Geometry: final body of the model. Coordinates: model frame, mm. A direction names the side the tool comes from. Give positions to 0.01 mm unless a question says otherwise; leave off trailing zeros. Loops run counter-clockwise (first coordinate to the right, second up) from the corner with the lowest first, then second, coordinate; pieces in that order, holes last. Notation, with made-up numbers: (70.25, -1) -> (115.25, -1) arc R25 ccw to (115.25, 17) -> close; hole circle Ø8 at (-1.75, 16.5). An arc over 180 degrees is marked (long way). Answer in a Markdown table with one row per item. Add a question column.
1) Line query: line 1 (X direction, y = 9, z = 0); line 2 (Y direction, x = -2.75, z = 5); line 3 (X direction, y = 25.75, z = 2.25). Output: solid intervals per line, ascending. Write a range as from..to.
2) Access query for faces 5 (the flat face through (-1, 27, -2)), 6 (the cylindrical face through (-3.905, 16.86, -0.867)). Directions: +Z, -Z, +X, -X, +Y, -Y. A direction counts if a zero-diameter tool reaches every point of the face in a straight line with its end or side. Return the directions, or none.
3) Section query B-B (y = 11.5). Return the cut outline in (x, z).
4) First-contact query: P1, Ø3, axis at y = 22, z = 1, coming from the +X side; P2, Ø1.5, axis at x = -5, y = 9.5, coming from the +Z side; P3, Ø5, axis at y = 14, z = 2, coming from the -X side; P4, Ø4, axis at x = 3.5, y = 22.5, coming from the +Z side. Flat tips, straight axial feed; report the tip coordinate or a pass-through.
5) Draft query along X for faces 1 (the flat face through (-4.956, 2.958, -2.915)), 2 (the flat face through (2, 6, -5)), 3 (the cylindrical face through (-2, 13, 0)), 4 (the flat face through (5.003, 2.958, -2.835)). Return one class per face: +X half, -X half, draft (parallel to the pull), parting line (faces both ways), or undercut.
6) Section query A-A (x = 0). Return the cut outline in (y, z).
```python
from build123d import *

# Parameters (mm, degrees)
SKETCH_1_R               = 4
EXTRUDE_2_DEPTH          = 27
SKETCH_1_5_R             = 4
EXTRUDE_3_DEPTH          = 6
FILLET_1_R               = 1
CUT_EXTRUDE_1_DEPTH      = 29.392707397
CUT_EXTRUDE_1_DEPTH_BACK = 29.392707397
SKETCH_2_R               = 2


with BuildPart() as part:
    # Sketch 1 → Extrude 2 (new body)
    with BuildSketch(Plane(origin=(0, 0, 0), x_dir=(1, 0, 0), z_dir=(0, 1, 0))):
        with Locations(Location((0, 0, 0), (0, 0, 270))):
            Circle(SKETCH_1_R)
    extrude(amount=EXTRUDE_2_DEPTH)

    # Sketch 1_5 → Extrude 3 (add)
    with BuildSketch(Plane(origin=(0, 0, 0), x_dir=(1, 0, 0), z_dir=(0, 1, 0))):
        Polygon((6.639528096, 0), (3.319764048, 5.75), (-3.319764048, 5.75), (-6.639528096, 0), (-3.319764048, -5.75), (3.319764048, -5.75), align=None)
        with Locations(Location((0, 0, 0), (0, 0, 270))):
            Circle(SKETCH_1_5_R, mode=Mode.SUBTRACT)
    extrude(amount=EXTRUDE_3_DEPTH)

    # Fillet 1
    fillet_1_edges = [part.edges().sort_by_distance(p)[0] for p in [
        (0, 6, -4),
    ]]
    fillet(fillet_1_edges, radius=FILLET_1_R)

    # Sketch 2 → Cut-Extrude 1 (cut, two sides: drawn at the far end of the back side and taken through both)
    with BuildSketch(Plane(origin=(0, 0, 0), x_dir=(1, 0, 0), z_dir=(0, 1, 0)).offset(-CUT_EXTRUDE_1_DEPTH_BACK)):
        with Locations(Location((0, 0, 0), (0, 0, 270))):
            Circle(SKETCH_2_R)
    extrude(amount=CUT_EXTRUDE_1_DEPTH + CUT_EXTRUDE_1_DEPTH_BACK, mode=Mode.SUBTRACT)


solid = part.part
```
Evaluation:
| question | item | result |
|---|---|---|
| 1 | line 1 | -4..-2, 2..4 |
| 1 | line 2 | 0..6 |
| 1 | line 3 | -3.31..3.31 |
| 2 | face 5 | +Z, -Z, +X, -X, +Y |
| 2 | face 6 | +Y |
| 3 | outline | circle Ø8 at (0, 0); hole circle Ø4 at (0, 0) |
| 4 | P1 | x = 4 |
| 4 | P2 | through |
| 4 | P3 | x = -4 |
| 4 | P4 | z = 3.71 |
| 5 | face 1 | -X half |
| 5 | face 2 | draft |
| 5 | face 3 | undercut |
| 5 | face 4 | +X half |
| 6 | outline | (0, -5.75) -> (6, -5.75) -> (6, -5) arc R1 cw to (7, -4) -> (27, -4) -> (27, -2) -> (0, -2) -> close; (0, 2) -> (27, 2) -> (27, 4) -> (7, 4) arc R1 cw to (6, 5) -> (6, 5.75) -> (0, 5.75) -> close |
